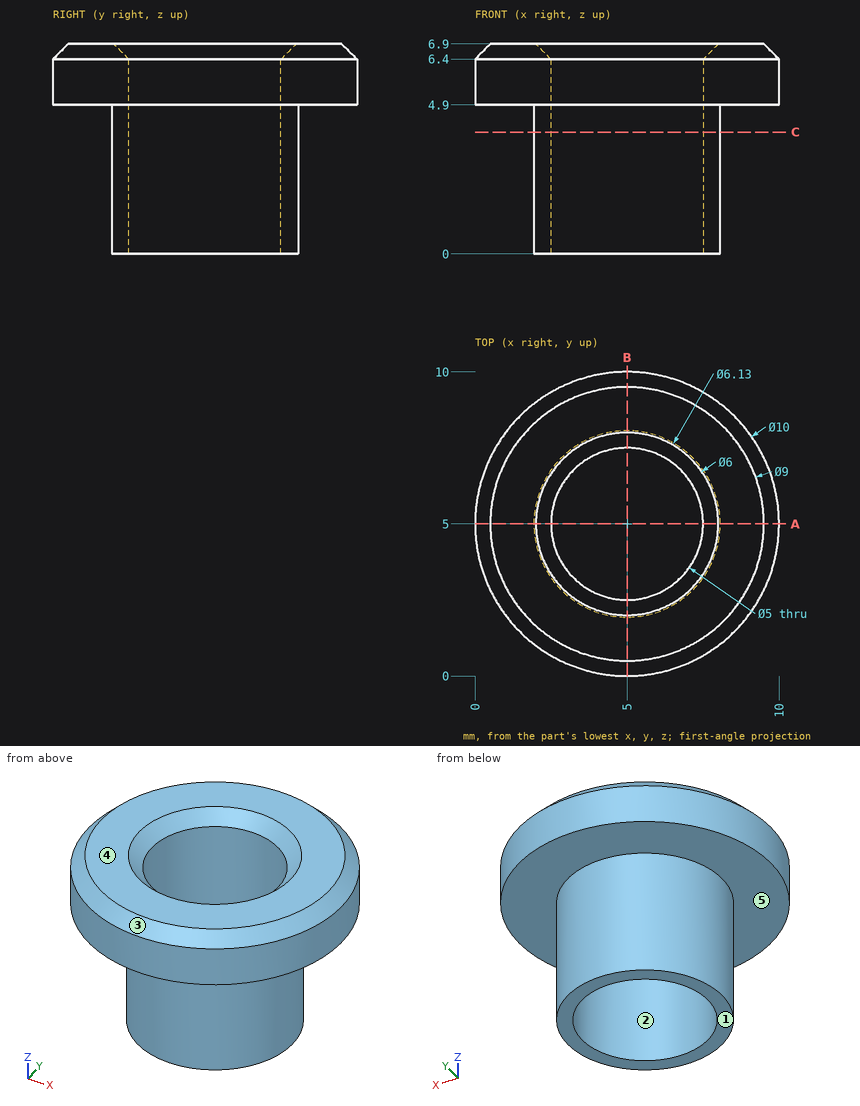
For this review, use the dimensioned drawing (mm, ordinates from the lowest corner) and the shaded views. A direction names the side the tool comes from. Coordinates: 2 decimals unless noted, no trailing zeros. Loops run counter-clockwise (first coordinate to the right, second up) from the corner with the lowest first, then second, coordinate; pieces in that order, holes last. Notation, with made-up numbers: (26, -38) -> (50, -38) arc R34 cw to (50, 1) -> close; hole circle Ø9 at (-15.75, -12.75). An arc over 180 degrees is marked (long way). Return JSON: item names as keys, results as strings. Group by question number.
(1) To check wall thickness, follow L1, parallel to Y at x = 5, z = 2 (3 decimals); L2, parallel to X at y = 6, z = 5.5; L3, parallel to X at y = 4.75, z = 2.75. State the ranges of each line that lie inside material, in increasing order.
(2) Mouldability with a two-part tool opening along Y and no side actions: class the marked faces 1, 2 and 3 as pulls with the +Y half, pulls with the -Y half, needs draft (parallel to the pull), parting line crosses it, or undercut.
(3) Consider section C-C, the plane z = 4. Give the boundary of the cut face in (x, y) (3 decimals), plus the area to 3 significant figures.
(4) Tool access review of the marked faces 4 and 5: name each direction out of +Z, -Z, +X, -X, +Y, -Y from which nothing blocks a thin tool from reaching the whole face with its end or side.
(5) For pin 1 Ø1 at (x, z) = (4, 1) entering from -Y; pin 2 Ø4 at (x, z) = (3.5, 1) entering from +Y (3 decimals); pin 3 Ø2 at (y, z) = (9, 6) entering from +X, all flat-tipped, find the tip position at first contact; note any pin that passes through.
(6) Consider section A-A, the plane y = 5. Give the boundary of the cut face in (x, z) (3 decimals), plus the area to 3 significant figures.
Results below:
{
 "1": {"L1": "y = 1.935 to 2.5, 7.5 to 8.065", "L2": "x = 0.1 to 2.71, 7.29 to 9.9", "L3": "x = 1.95 to 2.51, 7.49 to 8.05"},
 "2": {"face 1": "needs draft", "face 2": "undercut", "face 3": "parting line crosses it"},
 "3": {"outline": "circle Ø6.13 at (5, 5); hole circle Ø5 at (5, 5)", "area": "9.88 mm2"},
 "4": {"face 4": "+Z, +X, -X, +Y, -Y", "face 5": "-Z"},
 "5": {"pin 1": "stops at y = 1.98", "pin 2": "stops at y = 8.065", "pin 3": "stops at x = 9"},
 "6": {"outline": "(0, 4.9) -> (1.935, 4.9) -> (1.935, 0) -> (2.5, 0) -> (2.5, 6.4) -> (2, 6.9) -> (0.5, 6.9) -> (0, 6.4) -> close; (7.5, 0) -> (8.065, 0) -> (8.065, 4.9) -> (10, 4.9) -> (10, 6.4) -> (9.5, 6.9) -> (8, 6.9) -> (7.5, 6.4) -> close", "area": "15.0 mm2"}
}
